```python
from build123d import *

# Parameters (mm, degrees)
SKETCH1_R           = 3.2385
SKETCH1_R_2         = 75
BOSS_EXTRUDE1_DEPTH = 2.54


with BuildPart() as part:
    # Sketch1 → Boss-Extrude1 (new body)
    with BuildSketch(Plane(origin=(0, 0, 0), x_dir=(1, 0, 0), z_dir=(0, 1, 0))):
        Polygon((123.825, 152.4), (123.825, 123.825), (152.4, 123.825), (152.4, -123.825), (123.825, -123.825), (123.825, -152.4), (-123.825, -152.4), (-123.825, -123.825), (-152.4, -123.825), (-152.4, 123.825), (-123.825, 123.825), (-123.825, 152.4), align=None)
        with Locations((76.2, 139.7)):
            Circle(SKETCH1_R, mode=Mode.SUBTRACT)
        with Locations((0, 139.7)):
            Circle(SKETCH1_R, mode=Mode.SUBTRACT)
        with Locations((-76.2, 139.7)):
            Circle(SKETCH1_R, mode=Mode.SUBTRACT)
        with Locations((-76.2, -139.7)):
            Circle(SKETCH1_R, mode=Mode.SUBTRACT)
        with Locations((0, -139.7)):
            Circle(SKETCH1_R, mode=Mode.SUBTRACT)
        with Locations((76.2, -139.7)):
            Circle(SKETCH1_R, mode=Mode.SUBTRACT)
        with Locations((139.7, -76.2)):
            Circle(SKETCH1_R, mode=Mode.SUBTRACT)
        with Locations((139.7, 0)):
            Circle(SKETCH1_R, mode=Mode.SUBTRACT)
        with Locations((139.7, 76.2)):
            Circle(SKETCH1_R, mode=Mode.SUBTRACT)
        with Locations((-139.7, 76.2)):
            Circle(SKETCH1_R, mode=Mode.SUBTRACT)
        with Locations((-139.7, 0)):
            Circle(SKETCH1_R, mode=Mode.SUBTRACT)
        with Locations((-139.7, -76.2)):
            Circle(SKETCH1_R, mode=Mode.SUBTRACT)
        Circle(SKETCH1_R_2, mode=Mode.SUBTRACT)
    extrude(amount=BOSS_EXTRUDE1_DEPTH)


solid = part.part
```
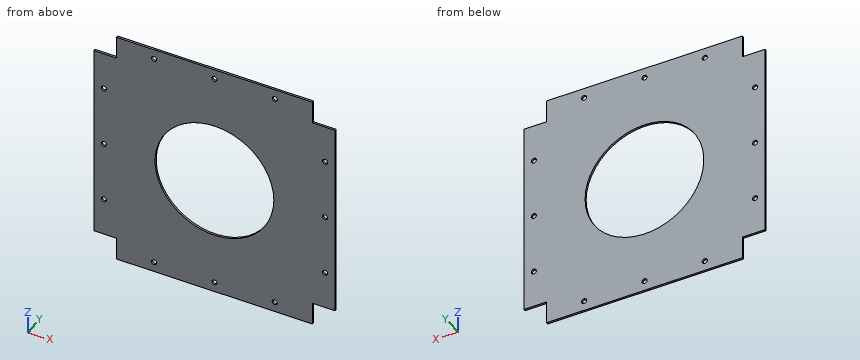
Geometry check sheet. Reference: the model listing, model coordinates, mm. Give positions to 0.01 mm unless a question says otherwise; leave off trailing zeros. Write each loop counter-clockwise with the first axis right and the second up, starting at its lowest first coordinate (ties: lowest second). Pieces come first, ordered by that corner, then holes. Notation, with made-up numbers: (-10, 54.25) -> (4, 54.25) arc R12 ccw to (4, 73.25) -> close; hole circle Ø9 at (-17, 64.5). An arc over 180 degrees is marked (long way). Use one line per item in the form item = value.
Item 1: Depth check by flat-ended pin: pin 1 Ø10.5 at (x, z) = (-76.2, -139.7) entering from -Y; pin 2 Ø0.8 at (y, z) = (1, 143.5) entering from +X (3 decimals). Enter the tip coordinate at first touch or a pass-through.
Results list:
pin_1 = 0
pin_2 = 123.825
Item 2: Sectioned sample at A-A on y = 1.15. Count the separate pieces of the cut face and the enclosed holes in it, plus the area to 3 significant figures.
Results list:
separate_pieces = 1
enclosed_holes = 13
area = 71,600 mm2
Item 3: Sectioned sample at D-D on x = 133. Enter the section's corners in (y, z) (3 decimals), plus the area to 3 significant figures.
Results list:
outline = (0, -123.825) -> (2.54, -123.825) -> (2.54, 123.825) -> (0, 123.825) -> close
area = 629 mm2
Item 4: Scan lines: line 1 (X direction, y = 1.6, z = 76.2); line 2 (X direction, y = 1.3, z = 0); line 3 (Z direction, x = -139.7, y = 1.4) (1 decimal). Record each from-to range of solid material in increasing order.
Results list:
line_1 = -152.4 to -142.94, -136.46 to 136.46, 142.94 to 152.4
line_2 = -152.4 to -142.94, -136.46 to -75, 75 to 136.46, 142.94 to 152.4
line_3 = -123.8 to -79.4, -73 to -3.2, 3.2 to 73, 79.4 to 123.8
Item 5: Sectioned sample at C-C on x = 17.5. Enter the section's corners in (y, z).
Results list:
outline = (0, -152.4) -> (2.54, -152.4) -> (2.54, -72.93) -> (0, -72.93) -> close; (0, 72.93) -> (2.54, 72.93) -> (2.54, 152.4) -> (0, 152.4) -> close
Item 6: Sectioned sample at B-B on z = -43. Enter the section's corners in (x, y), plus the area to 3 significant figures.
Results list:
outline = (-152.4, 0) -> (-61.45, 0) -> (-61.45, 2.54) -> (-152.4, 2.54) -> close; (61.45, 0) -> (152.4, 0) -> (152.4, 2.54) -> (61.45, 2.54) -> close
area = 462 mm2
